Verification items for the finished model (mm, model axes). A direction names the side the tool comes from. Round coordinates to 2 decimals unless told otherwise and drop trailing zeros. Write each loop counter-clockwise with the first axis right and the second up, starting at its lowest first coordinate (ties: lowest second). Pieces come first, ordered by that corner, then holes. Notation, with made-up numbers: (26.25, 57) - (71.25, 57) arc R23 cw to (71.25, 70) - close; hole circle Ø8 at (3, 18.25). An arc over 180 degrees is marked (long way). Answer as a JSON object with one key per item and string values.
```python
from build123d import *

# Parameters (mm, degrees)
F0_W      = 19
F0_H      = 19
F1_DEPTH  = 2
F4_DEPTH  = 9
F2_R      = 6
F5_DEPTH  = 17
F7_DEPTH  = 10
F10_R     = 1
F11_DEPTH = 20
F12_W     = 10
F12_H     = 4
F13_DEPTH = 4


# Not quite as in the source:
# - a feature of the source that left no trace in its solid (it failed there, or was rolled back) is left out
# - a feature names something its author has since deleted; it is built from what else it names


with BuildPart() as f1:
    # F0 (on Front) → F1 (new body)
    with BuildSketch(Plane.XZ):
        Rectangle(F0_W, F0_H)
    extrude(amount=F1_DEPTH)

    # F3 (on face) → F4 (join)
    with BuildSketch(Plane.XZ.offset(2)):
        with BuildLine():
            Line((-5.5251262658, 6.9393398282), (-6.5023238038, 7.9165373661))
            ThreePointArc((-6.5023238038, 7.9165373661), (-6.9102307697, 9.0307293654), (-8, 9.5))
            ThreePointArc((-8, 9.5), (-9.0606601718, 9.0606601718), (-9.5, 8))
            ThreePointArc((-9.5, 8), (-9.0307293654, 6.9102307697), (-7.9165373661, 6.5023238038))
            Line((-7.9165373661, 6.5023238038), (-6.9393398282, 5.5251262658))
            Line((-6.9393398282, 5.5251262658), (-6.9393398282, -6.9393398282))
            Line((-6.9393398282, -6.9393398282), (5.5251262658, -6.9393398282))
            Line((5.5251262658, -6.9393398282), (6.5023238038, -7.9165373661))
            ThreePointArc((6.5023238038, -7.9165373661), (6.9102307697, -9.0307293654), (8, -9.5))
            ThreePointArc((8, -9.5), (9.0606601718, -9.0606601718), (9.5, -8))
            ThreePointArc((9.5, -8), (9.0307293654, -6.9102307697), (7.9165373661, -6.5023238038))
            Line((7.9165373661, -6.5023238038), (6.9393398282, -5.5251262658))
            Line((6.9393398282, -5.5251262658), (6.9393398282, 6.9393398282))
            Line((6.9393398282, 6.9393398282), (-5.5251262658, 6.9393398282))
        make_face()
    extrude(amount=F4_DEPTH)

    # F2 (on face) → F5 (join)
    with BuildSketch(Plane.XZ.offset(2)):
        Circle(F2_R)
    extrude(amount=F5_DEPTH)

    # F6 (on Right) → F7 (join, symmetric)
    with BuildSketch(Plane.YZ):
        with BuildLine():
            ThreePointArc((-7, 2.2071067812), (-7.1464466094, 2.5606601718), (-7.5, 2.7071067812))
            Line((-7.5, 2.7071067812), (-10.5, 2.7071067812))
            ThreePointArc((-10.5, 2.7071067812), (-10.8535533906, 2.5606601718), (-11, 2.2071067812))
            Line((-11, 2.2071067812), (-11, -0.7928932188))
            ThreePointArc((-11, -0.7928932188), (-10.8535533906, -1.1464466094), (-10.5, -1.2928932188))
            Line((-10.5, -1.2928932188), (-7.5, -1.2928932188))
            ThreePointArc((-7.5, -1.2928932188), (-7.1464466094, -1.1464466094), (-7, -0.7928932188))
            Line((-7, -0.7928932188), (-7, 2.2071067812))
        make_face()
    extrude(amount=F7_DEPTH, both=True)

    # F10 (on face) → F11 (cut, symmetric)
    with BuildSketch(Plane.YZ.offset(6.9393398282)):
        with Locations((-9, 0.7071067812)):
            Circle(F10_R)
    extrude(amount=F11_DEPTH, both=True, mode=Mode.SUBTRACT)

    # F12 (on face) → F13 (join)
    with BuildSketch(Plane(origin=(0, 0, 0), x_dir=(-1, 0, 0), z_dir=(0, 1, 0))):
        with Locations((-4.5, 7.5)):
            Rectangle(F12_W, F12_H)
    extrude(amount=F13_DEPTH)


solid = f1.part
```
1. Go/stop test with flat-tipped pins: pin 1 (0.9 mm diameter, centred on x = 8, y = -9, fed in from +Z); pin 2 (8 mm diameter, centred on x = -5, y = -14, fed in from +Z); pin 3 (1.2 mm diameter, centred on y = 1, z = 8, fed in from -X). Record where each tip stops, or that it passes through.
Completed:
{"pin 1": "stops at z = 2.71", "pin 2": "stops at z = 9.46", "pin 3": "stops at x = -0.5"}
2. Cross-section at D-D (x = 0). Record the boundary of the cut face in (y, z).
Completed:
{"outline": "(-19, -6) - (-11, -6) - (-11, -6.94) - (-2, -6.94) - (-2, -9.5) - (0, -9.5) - (0, 5.5) - (4, 5.5) - (4, 9.5) - (-2, 9.5) - (-2, 6.94) - (-11, 6.94) - (-11, 6) - (-19, 6) - close; hole circle Ø2 at (-9, 0.71)"}
3. Cross-section at B-B (z = 0). Record the boundary of the cut face in (x, y), plus the area to 3 significant figures.
Completed:
{"outline": "(-10, -11) - (-6, -11) - (-6, -19) - (6, -19) - (6, -11) - (10, -11) - (10, -9.71) - (-10, -9.71) - close; (-10, -8.29) - (10, -8.29) - (10, -7) - (6.94, -7) - (6.94, -2) - (9.5, -2) - (9.5, 0) - (-9.5, 0) - (-9.5, -2) - (-6.94, -2) - (-6.94, -7) - (-10, -7) - close", "area": "255 mm^2"}
4. Cross-section at A-A (y = -9). Record the boundary of the cut face in (x, z).
Completed:
{"outline": "(-10, -1.29) - (-6.94, -1.29) - (-6.94, -6.94) - (5.53, -6.94) - (6.5, -7.92) arc R1.5 ccw (long way) to (7.92, -6.5) - (6.94, -5.53) - (6.94, -1.29) - (10, -1.29) - (10, -0.29) - (-10, -0.29) - close; (-10, 1.71) - (10, 1.71) - (10, 2.71) - (6.94, 2.71) - (6.94, 6.94) - (-5.53, 6.94) - (-6.5, 7.92) arc R1.5 ccw (long way) to (-7.92, 6.5) - (-6.94, 5.53) - (-6.94, 2.71) - (-10, 2.71) - close"}
5. Cross-section at C-C (x = 2.75). Record the boundary of the cut face in (y, z), plus the area to 3 significant figures.
Completed:
{"outline": "(-19, -5.33) - (-11, -5.33) - (-11, -6.94) - (-2, -6.94) - (-2, -9.5) - (0, -9.5) - (0, 5.5) - (4, 5.5) - (4, 9.5) - (-2, 9.5) - (-2, 6.94) - (-11, 6.94) - (-11, 5.33) - (-19, 5.33) - close; hole circle Ø2 at (-9, 0.71)", "area": "261 mm^2"}
6. Mould release check, pull along Y, two halves, no side actions. Record for faces 1 (the face through (-9.2, -2, 9.14)), 2 (the face through (-8, -7, 1)), 3 (the face through (-6, -15, 0)): released by +Y, released by -Y, zero draft, split by the parting line, or undercut.
Completed:
{"face 1": "released by -Y", "face 2": "undercut", "face 3": "zero draft"}
7. Access from +Z, -Z, +X, -X, +Y, -Y to the whole of each face (thin tool, end or side, straight path). Record for faces 4 (the face through (6.007, -6.437, -7.421)), 5 (the face through (-7.435, -6.437, 6.021)), 6 (the face through (-5, -11, 4)), 7 (the face through (7.435, -6.437, -6.021)), 8 (the face through (9.2, -2, -9.2)).
Completed:
{"face 4": "-Z, -X, -Y", "face 5": "-X, -Y", "face 6": "-Y", "face 7": "+X, -Y", "face 8": "-Z, +X, -Y"}
8. Material ranges on probe 1 along Y at (x, z) = (7.5, 1.75); probe 2 along Y at (x, z) = (-1.5, -8.5); probe 3 along Z at (x, y) = (-4.75, -9), recorded low to high. Write a range as from..to.
Completed:
{"probe 1": "y = -11..-7, -2..0", "probe 2": "y = -2..0", "probe 3": "z = -6.94..-0.29, 1.71..6.94"}
